For this review, take the finished solid that the model builds, in its own axes (mm). Coordinates: 2 decimals unless noted, no trailing zeros. Loops run counter-clockwise (first coordinate to the right, second up) from the corner with the lowest first, then second, coordinate; pieces in that order, holes last. Notation, with made-up numbers: (48.5, 63.5) -> (64.5, 63.5) arc R36 cw to (64.5, 97.5) -> close; hole circle Ø2 at (-27, -14.5). An arc over 180 degrees is marked (long way). Use a Markdown table: item, result.
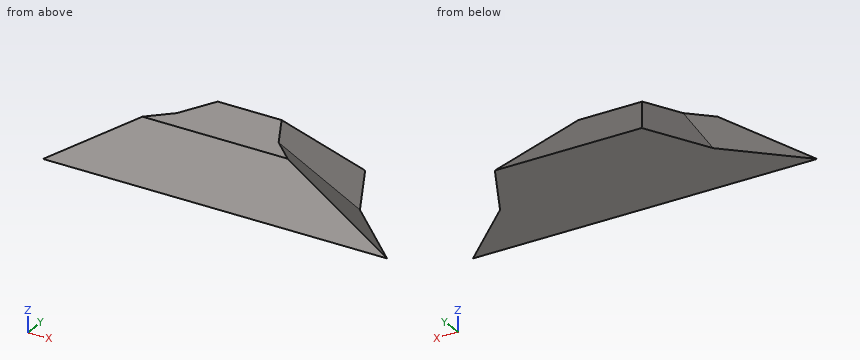
from build123d import *

# Parameters (mm, degrees)
F1_DEPTH = 20
F2_SIZE  = 19.99999


# Not quite as in the source:
# - a fillet or chamfer is up to 0.001 mm smaller than in the source, because OpenCascade refuses the exact size


with BuildPart() as f1:
    # F0 (on Top) → F1 (new body)
    with BuildSketch(Plane.XY):
        Polygon((-30.9781403543, -6.75), (-50, -25), (50, -25), (30.9781403543, -6.75), (21.3486810742, 11.5), (-21.3486810742, 11.5), align=None)
    extrude(amount=F1_DEPTH)

    # F2 (size 20 in the source; OpenCascade refuses exactly that, so slightly less here)
    f2_edges = [f1.edges().sort_by_distance(p)[0] for p in [
        (0, 11.5, 20),
        (26.163411, 2.375, 20),
        (40.48907, -15.875, 20),
        (-40.48907, -15.875, 20),
        (-26.163411, 2.375, 20),
    ]]
    chamfer(f2_edges, length=F2_SIZE)


solid = f1.part
(1) For pin 1 Ø4 at (x, z) = (31.5, 10) entering from +Y; pin 2 Ø3 at (y, z) = (-11.5, 11.5) entering from -X; pin 3 Ø3 at (y, z) = (-3, 12.5) entering from +X, all flat-tipped, find the tip position at first contact; note any pin that passes through.
Found:
| item | result |
|---|---|
| pin 1 | stops at y = -17.74 |
| pin 2 | stops at x = -22.35 |
| pin 3 | stops at x = 16.74 |
(2) Take a section at B-B on z = 13.25. Write out the cut boundary in (x, y), plus the area to 3 significant figures.
Found:
| item | result |
|---|---|
| outline | (-30.86, -25) -> (30.86, -25) -> (20.26, -14.83) -> (13.36, -1.75) -> (-13.36, -1.75) -> (-20.26, -14.83) -> close |
| area | 960 mm^2 |
(3) For line 1 along Z through (x, y) = (12.5, 7.5); line 2 along X through (y, z) = (-21, 9); line 3 along X through (y, z) = (-14, 18.5), list the stretches that pass through material, from the lowest coordinate up.
Found:
| item | result |
|---|---|
| line 1 | z = 0 to 4 |
| line 2 | x = -32.83 to 32.83 |
| line 3 | x = -13.89 to 13.89 |
